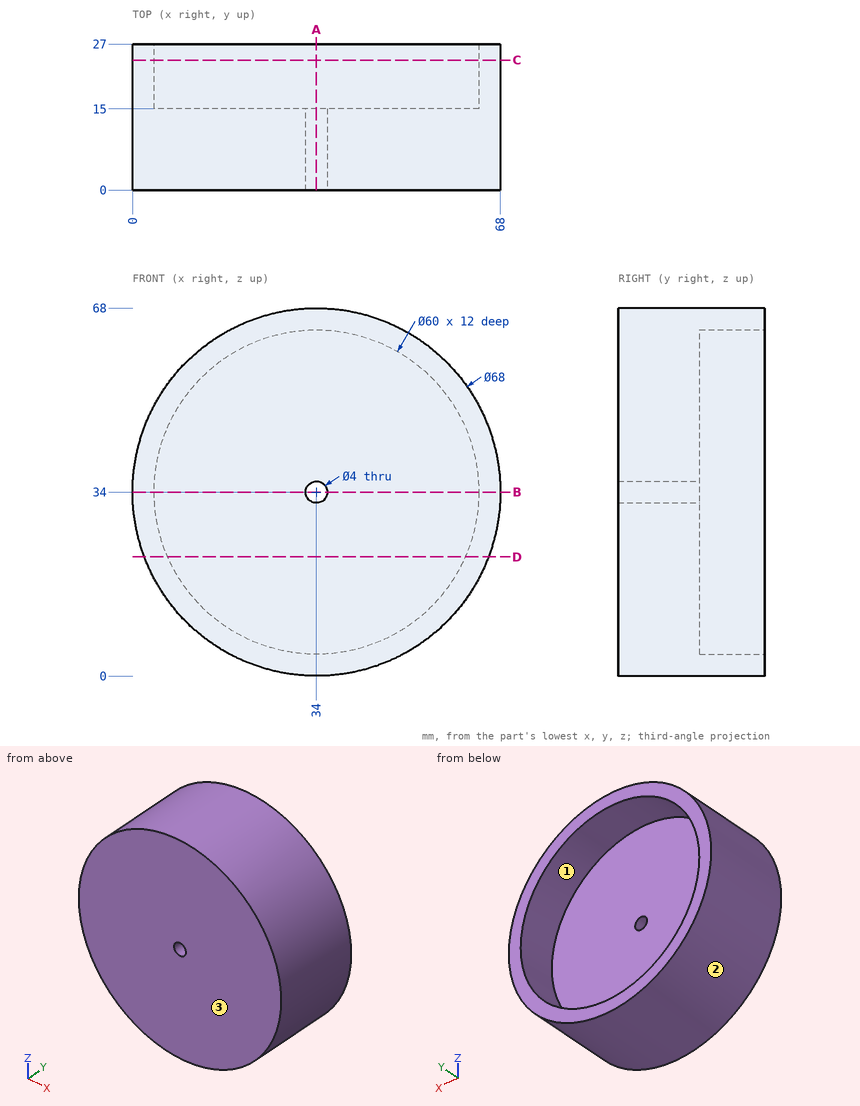
Check sheet for the drawn part. Datum: minimum x, y, z corner. Units: mm. Round coordinates to 2 decimals unless told otherwise and drop trailing zeros. Loops run counter-clockwise (first coordinate to the right, second up) from the corner with the lowest first, then second, coordinate; pieces in that order, holes last. Notation, with made-up numbers: (62.25, 5) -> (78.25, 5) arc R34 cw to (78.25, 38) -> close; hole circle Ø11 at (-15.75, 46.5). An arc over 180 degrees is marked (long way). Put each result on its own line as item: value. Start each with the question number.
1. Draft check along X on the marked faces 1, 2 and 3. Enter one of: +X half, -X half, draft (parallel to the pull), parting line (faces both ways), or undercut.
2. Section check A-A (x = 34). Enter the section's corners in (y, z).
3. Gauge pin test, flat ends, axial feed: pin 1 (3 mm diameter, centred on x = 26, y = 12.5, fed in from +Z); pin 2 (1.5 mm diameter, centred on x = 44, y = 9.5, fed in from +Z); pin 3 (3 mm diameter, centred on x = 48.5, z = 56.5, fed in from +Y). Record the tip position at first contact, or that the pin passes through.
4. Scan lines: probe 1 along Z at (x, y) = (34, 7.25); probe 2 along X at (y, z) = (18, 35); probe 3 along Z at (x, y) = (34, 21.5). Record each from-to range of solid material in increasing order.
5. Section check D-D (z = 22). Enter the section's corners in (x, y), plus the area to 3 significant figures.
6. Section check B-B (z = 34). Enter the section's corners in (x, y).
7. Section check C-C (y = 24). Enter the section's corners in (x, z).
Findings:
1. face 1: undercut
1. face 2: parting line
1. face 3: draft
2. outline: (0, 0) -> (27, 0) -> (27, 4) -> (15, 4) -> (15, 32) -> (0, 32) -> close; (0, 36) -> (15, 36) -> (15, 64) -> (27, 64) -> (27, 68) -> (0, 68) -> close
3. pin 1: stops at z = 67.37
3. pin 2: stops at z = 66.72
3. pin 3: stops at y = 15
4. probe 1: z = 0 to 32, 36 to 68
4. probe 2: x = 0.01 to 4.02, 63.98 to 67.99
4. probe 3: z = 0 to 4, 64 to 68
5. outline: (2.19, 0) -> (65.81, 0) -> (65.81, 27) -> (61.5, 27) -> (61.5, 15) -> (6.5, 15) -> (6.5, 27) -> (2.19, 27) -> close
5. area: 1,060 mm^2
6. outline: (0, 0) -> (32, 0) -> (32, 15) -> (4, 15) -> (4, 27) -> (0, 27) -> close; (36, 0) -> (68, 0) -> (68, 27) -> (64, 27) -> (64, 15) -> (36, 15) -> close
7. outline: circle Ø68 at (34, 34); hole circle Ø60 at (34, 34)
